The listing builds one solid part. Answer for the finished solid, in the listing's coordinates (mm). Face numbers are marked on the shaded views. A direction names the side the tool comes from. Coordinates: 2 decimals unless noted, no trailing zeros. Write each loop counter-clockwise with the first axis right and the second up, starting at its lowest first coordinate (ties: lowest second). Pieces come first, ordered by that corner, then holes. Notation, with made-up numbers: M 51.5,25.5 L 77.5,25.5 A18 ccw 77.5,46.5 Z; hole C 28,-15 d5. An arc over 180 degrees is marked long. Put each result on its own line as item: value. Start each with the question number.
```python
from build123d import *

# Parameters (mm, degrees)
F1_DEPTH = 25.4
F2_DEPTH = 50.8


with BuildPart() as f1:
    # F0 (on Top) → F1 (new body)
    with BuildSketch(Plane.XY):
        Polygon((80.641053, 41.950212), (29.841053, 16.550212), (29.841053, -8.849788), (80.641053, -34.249788), align=None)
    extrude(amount=F1_DEPTH)

    # F0 (on Top) → F2 (join)
    with BuildSketch(Plane.XY):
        Polygon((29.841053, 41.950212), (-71.758947, 41.950212), (-71.758947, -34.249788), (29.841053, -34.249788), (29.841053, -8.849788), (29.841053, 16.550212), align=None)
    extrude(amount=F2_DEPTH)


solid = f1.part
```
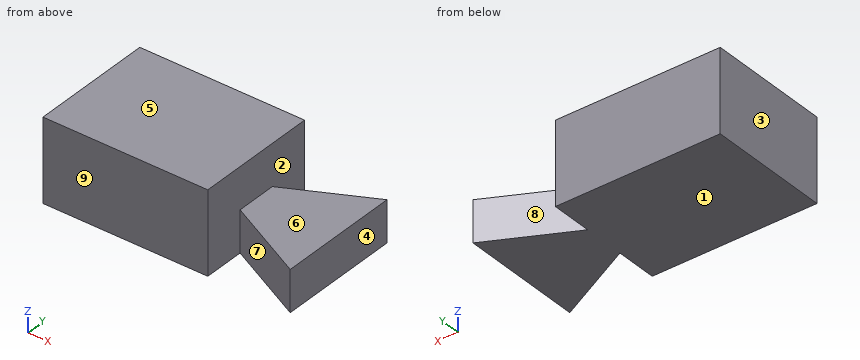
1) Given pin 1 Ø10 at (y, z) = (10, 31.5) entering from +X, flat-ended and moving along its own axis, determine where the tip first touches the part or whether it passes through.
2) Straight lines are drawn through the part: probe 1 along X at (y, z) = (7, 26); probe 2 along X at (y, z) = (34.5, 6); probe 3 along X at (y, z) = (-13.5, 2). For each, find the intervals that lie inside material, in ascending order.
3) A cutting plane is placed at D-D on x = 32.5. Write down the section's boundary in (y, z).
4) A cutting plane is placed at B-B on z = 13. Write down the section's boundary in (x, y).
5) For the marked faces 5, 6, 7, 8 and 9, determine the directions among +Z, -Z, +X, -X, +Y, -Y from which every point of the face is accessible in a straight line to the end or side of a thin tool.
6) A cutting plane is placed at C-C on y = -22. Write down the section's boundary in (x, z).
7) A cutting plane is placed at A-A on y = 22. Write down the section's boundary in (x, z), then the cut area to 3 significant figures.
8) Determine the mould class of the marked faces 1, 2, 3 and 4 for opening direction X: +X half, -X half, draft (parallel to the pull), parting line (faces both ways), or undercut.
Answers follow:
1. pin 1: stops at x = 29.84
2. probe 1: x = -71.76 to 29.84
2. probe 2: x = -71.76 to 29.84, 65.74 to 80.64
2. probe 3: x = -71.76 to 29.84, 39.14 to 80.64
3. outline: M -10.18,0 L 17.88,0 L 17.88,25.4 L -10.18,25.4 Z
4. outline: M -71.76,-34.25 L 29.84,-34.25 L 29.84,-8.85 L 80.64,-34.25 L 80.64,41.95 L 29.84,16.55 L 29.84,41.95 L -71.76,41.95 Z
5. face 5: +Z, +X, -X, +Y, -Y
5. face 6: +Z, +X, +Y, -Y
5. face 7: +Z, -Z, -Y
5. face 8: +Z, -Z, +Y
5. face 9: +Z, -Z, +X, -X, -Y
6. outline: M -71.76,0 L 29.84,0 L 29.84,50.8 L -71.76,50.8 Z; M 56.14,0 L 80.64,0 L 80.64,25.4 L 56.14,25.4 Z
7. outline: M -71.76,0 L 29.84,0 L 29.84,50.8 L -71.76,50.8 Z; M 40.74,0 L 80.64,0 L 80.64,25.4 L 40.74,25.4 Z
7. area: 6,170 mm²
8. face 1: draft
8. face 2: undercut
8. face 3: -X half
8. face 4: +X half
